Answer from the drawing. Dimensions are ordinates in mm from the lowest x, y and z of the part. A direction names the side the tool comes from. Give positions to 0.01 mm unless a question says otherwise; leave off trailing zeros. Loops run counter-clockwise (first coordinate to the right, second up) from the corner with the lowest first, then second, coordinate; pieces in that order, holes last. Notation, with made-up numbers: (13, 69.5) - (18, 69.5) arc R30 ccw to (18, 97.5) - close; hole circle Ø8 at (43, 72). An arc over 180 degrees is marked (long way). Put each result on its own line as item: value. Start each with the question number.
1. For the marked faces 1, 2, 3 and 4, determine the directions among +Z, -Z, +X, -X, +Y, -Y from which every point of the face is accessible in a straight line to the end or side of a thin tool.
2. A cutting plane is placed at A-A, the plane z = 33.25. Determine the outline of the cut face in (x, y).
3. Given pin 1 Ø5 at (x, y) = (18, 18.5) entering from -Z; pin 2 Ø4.5 at (x, z) = (52, 11.9) entering from +Y; pin 3 Ø6 at (x, z) = (51, 25) entering from -Y; pin 4 Ø8.5 at (x, y) = (55.5, 10.5) entering from -Z, each flat-ended and moving along its own axis, determine where each tip first touches the part or whether it passes through.
4. A cutting plane is placed at C-C, the plane x = 30.5. Determine the outline of the cut face in (y, z).
5. A cutting plane is placed at D-D, the plane z = 17. Determine the outline of the cut face in (x, y), plus the area to 3 significant figures.
6. A cutting plane is placed at B-B, the plane y = 6.5. Determine the outline of the cut face in (x, z), plus the area to 3 significant figures.
7. Consider L1, parallel to X at y = 21.6, z = 11.9; L2, parallel to Z at x = 12, y = 21.35; L3, parallel to Z at x = 13, y = 21.95. Determine where each line is inside the solid, lowest interval first. Write a range as from..to.
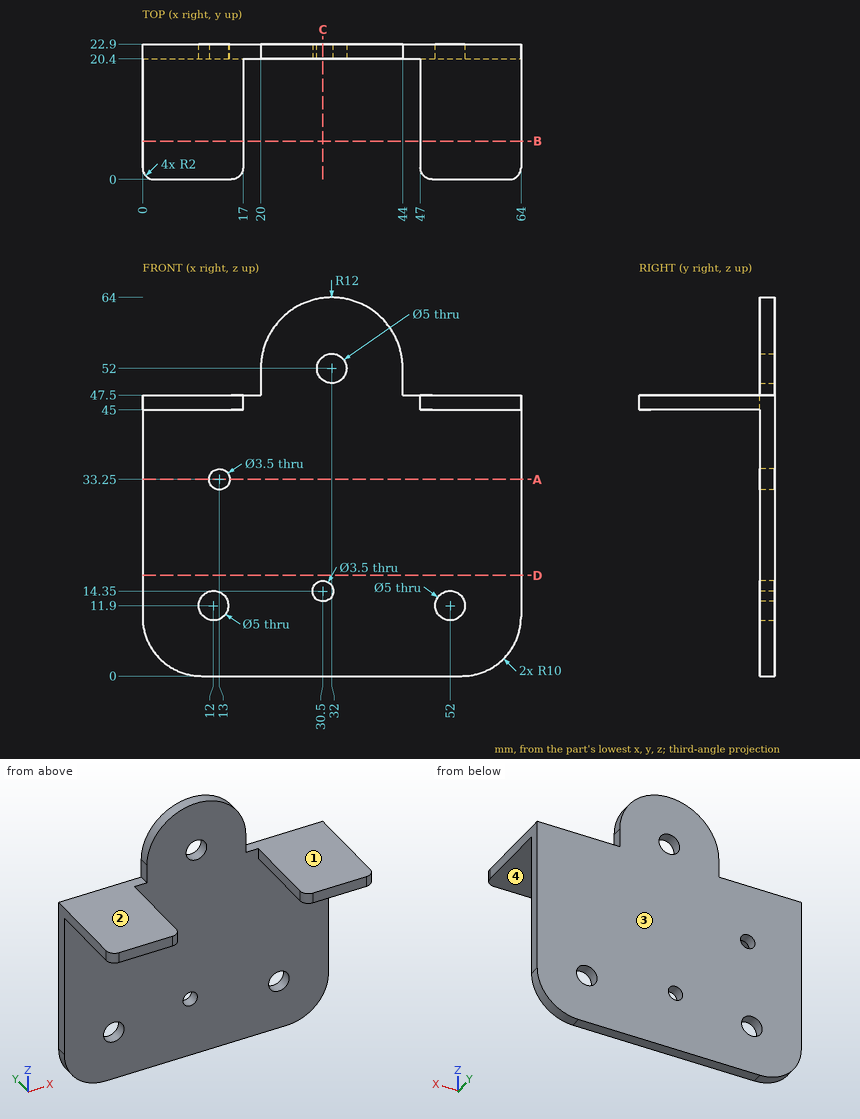
Return value:
1. face 1: +Z, +X, +Y, -Y
1. face 2: +Z, -X, +Y, -Y
1. face 3: +Z, -Z, +X, -X, +Y
1. face 4: -Z, +X, -X, -Y
2. outline: (0, 20.4) - (11.25, 20.4) - (11.25, 22.9) - (0, 22.9) - close; (14.75, 20.4) - (64, 20.4) - (64, 22.9) - (14.75, 22.9) - close
3. pin 1: stops at z = 0
3. pin 2: passes through
3. pin 3: stops at y = 20.4
3. pin 4: stops at z = 45
4. outline: (20.4, 0) - (22.9, 0) - (22.9, 12.6) - (20.4, 12.6) - close; (20.4, 16.1) - (22.9, 16.1) - (22.9, 50) - (20.4, 50) - close; (20.4, 54) - (22.9, 54) - (22.9, 63.91) - (20.4, 63.91) - close
5. outline: (0, 20.4) - (64, 20.4) - (64, 22.9) - (0, 22.9) - close
5. area: 160 mm2
6. outline: (0, 45) - (17, 45) - (17, 47.5) - (0, 47.5) - close; (47, 45) - (64, 45) - (64, 47.5) - (47, 47.5) - close
6. area: 85.0 mm2
7. L1: x = 0..9.5, 14.5..49.5, 54.5..64
7. L2: z = 0..9.4, 14.4..31.81, 34.69..47.5
7. L3: z = 0..9.61, 14.19..31.5, 35..47.5
